Source: CAD feature listing. Evaluate the final solid. Frame: model axes, mm. A direction names the side the tool comes from. Coordinates: 2 decimals unless noted, no trailing zeros. Write each loop counter-clockwise with the first axis right and the second up, starting at its lowest first coordinate (ties: lowest second). Pieces come first, ordered by that corner, then holes. Notation, with made-up numbers: M 20,85.25 L 35,85.25 A13 ccw 35,98.25 Z; hole C -7.5,71.5 d3. An arc over 180 degrees is marked long. Write item = value, one per line. Start each with the question number.
1. Section query A-A (x = 48.5). Output: boundary loops of the cut face in (y, z), then the cut area to 3 significant figures.
2. Line query: line 1 along Y through (x, z) = (-107, 0.3); line 2 along X through (y, z) = (6, 0.3); line 3 along Y through (x, z) = (-23, 0.65). Output: solid intervals per line, ascending.
3. Section query C-C (z = 0.75). Give the number of separate pieces and of enclosed holes in the cut face, then the cut area to 3 significant figures.
4. Section query B-B (x = 107). Output: boundary loops of the cut face in (y, z).
5. Section query D-D (y = 11.5). Output: boundary loops of the cut face in (x, z), then the cut area to 3 significant figures.
6. Access query for faces 3 (the face through (-2, 1, 1)), 4 (the face through (29, -0.16, 0.51)). Directions: +Z, -Z, +X, -X, +Y, -Y. A direction counts if a zero-diameter tool reaches every point of the face in a straight line with its end or side. Return the directions, or none.
7. Pull-direction query (X, two-part tool) for faces 1 (the face through (105.415, 33.453, 0.493)), 2 (the face through (-2, 1, 0)); classes: pulls with the +X half, pulls with the -X half, needs draft (parallel to the pull), parting line crosses it, or undercut.
```python
from build123d import *

# Parameters (mm, degrees)
SKETCH_1_W          = 228
SKETCH_1_H          = 84
SKETCH_1_R          = 2.15
EXTRUDE_1_DEPTH     = 1
SKETCH_4_R          = 1.6
SKETCH_4_W          = 14.464145402
SKETCH_4_H          = 14
CUT_EXTRUDE_2_DEPTH = 1
SKETCH_5_R          = 1.7
SKETCH_5_R_2        = 3
SKETCH_5_R_3        = 2.5
CUT_EXTRUDE_3_DEPTH = 10


with BuildPart() as part:
    # Эскиз1 → Вытянуть1 (new body)
    with BuildSketch(Plane.XY):
        Rectangle(SKETCH_1_W, SKETCH_1_H)
        with Locations((107, 32)):
            Circle(SKETCH_1_R, mode=Mode.SUBTRACT)
        with Locations(Location((-107, 32, 0), (0, 0, 180))):
            Circle(SKETCH_1_R, mode=Mode.SUBTRACT)
        with Locations((-107, -32)):
            Circle(SKETCH_1_R, mode=Mode.SUBTRACT)
        with Locations(Location((107, -32, 0), (0, 0, 180))):
            Circle(SKETCH_1_R, mode=Mode.SUBTRACT)
    extrude(amount=EXTRUDE_1_DEPTH)

    # Эскиз4 → Вырез-Вытянуть2 (cut)
    with BuildSketch(Plane.XY.offset(1)):
        with Locations((19, 2)):
            Circle(SKETCH_4_R)
        with Locations((84, 2)):
            Circle(SKETCH_4_R)
        with Locations((-84, 2)):
            Circle(SKETCH_4_R)
        with Locations((-35, 2)):
            Circle(SKETCH_4_R)
        with BuildLine():
            Line((36.5, 7.5), (66.5, 7.5))
            ThreePointArc((66.5, 7.5), (74, 0), (66.5, -7.5))
            Line((66.5, -7.5), (36.5, -7.5))
            ThreePointArc((36.5, -7.5), (29, 0), (36.5, 7.5))
        make_face()
        with BuildLine():
            Line((-67, 7.5), (-52, 7.5))
            ThreePointArc((-52, 7.5), (-44.5, 0), (-52, -7.5))
            Line((-52, -7.5), (-67, -7.5))
            ThreePointArc((-67, -7.5), (-74.5, 0), (-67, 7.5))
        make_face()
        with Locations((-111.232072701, 7)):
            Rectangle(SKETCH_4_W, SKETCH_4_H)
    extrude(amount=-CUT_EXTRUDE_2_DEPTH, mode=Mode.SUBTRACT)

    # Эскиз5 → Вырез-Вытянуть3 (cut)
    with BuildSketch(Plane.XY.offset(1)):
        with Locations((-53, 32)):
            Circle(SKETCH_5_R)
        with Locations((37, 32)):
            Circle(SKETCH_5_R)
        with Locations((-13, 32)):
            Circle(SKETCH_5_R_2)
        with Locations((-23, 32)):
            Circle(SKETCH_5_R_2)
        with Locations((-33, 32)):
            Circle(SKETCH_5_R_2)
        with Locations((-43, 32)):
            Circle(SKETCH_5_R_2)
        with Locations((-1, -17)):
            Circle(SKETCH_5_R_3)
        with Locations((84, -17)):
            Circle(SKETCH_5_R_3)
        with Locations(Location((-3, 32, 0), (0, 0, 180))):
            Circle(SKETCH_5_R_2)
        with Locations(Location((7, 32, 0), (0, 0, 180))):
            Circle(SKETCH_5_R_2)
        with Locations(Location((17, 32, 0), (0, 0, 180))):
            Circle(SKETCH_5_R_2)
        with Locations(Location((27, 32, 0), (0, 0, 180))):
            Circle(SKETCH_5_R_2)
    extrude(amount=-CUT_EXTRUDE_3_DEPTH, mode=Mode.SUBTRACT)


solid = part.part
```
Results are:
q1.outline = M -42,0 L -7.5,0 L -7.5,1 L -42,1 Z; M 7.5,0 L 42,0 L 42,1 L 7.5,1 Z
q1.area = 69.0 mm^2
q2.line_1 = -42 to -34.15, -29.85 to 0, 14 to 29.85, 34.15 to 42
q2.line_2 = -104 to -71.5, -47.5 to 32, 71 to 114
q2.line_3 = -42 to 29, 35 to 42
q3.separate_pieces = 1
q3.enclosed_holes = 22
q3.area = 17,600 mm^2
q4.outline = M -42,0 L -34.15,0 L -34.15,1 L -42,1 Z; M -29.85,0 L 29.85,0 L 29.85,1 L -29.85,1 Z; M 34.15,0 L 42,0 L 42,1 L 34.15,1 Z
q5.outline = M -104,0 L 114,0 L 114,1 L -104,1 Z
q5.area = 218 mm^2
q6.face_3 = +Z, +X, -X, +Y, -Y
q6.face_4 = +Z, -Z
q7.face_1 = undercut
q7.face_2 = needs draft
